```python
from build123d import *

# Parameters (mm, degrees)
PAD_DEPTH       = 20
SKETCH001_R     = 2.6
POCKET_DEPTH    = 25.501
SKETCH002_R     = 5
POCKET001_DEPTH = 21.501
CHAMFER_SIZE    = 4
CHAMFER001_SIZE = 1.5


with BuildPart() as part:
    # Sketch → Pad (new body)
    with BuildSketch(Plane.XY):
        with BuildLine():
            ThreePointArc((-7.433034, 13), (7.5, 14), (-7.433034, 15))
            Line((-7.433034, 15), (-25.5, 15))
            Line((-25.5, 15), (-25.5, 19))
            Line((-25.5, 19), (-10.356158, 19))
            ThreePointArc((8.305538, 21.954121), (-1.798046, 25.358566), (-10.356158, 19))
            Line((25.5, 4), (8.305538, 21.954121))
            Line((25.5, 0), (25.5, 4))
            Line((-25.5, 0), (25.5, 0))
            Line((-25.5, 13), (-25.5, 0))
            Line((-7.433034, 13), (-25.5, 13))
        make_face()
    extrude(amount=PAD_DEPTH)

    # Sketch001 → Pocket (cut, through all)
    with BuildSketch(Plane.XZ):
        with Locations((-16.5, 10)):
            Circle(SKETCH001_R)
        with Locations((16.5, 10)):
            Circle(SKETCH001_R)
    extrude(amount=-POCKET_DEPTH, mode=Mode.SUBTRACT)

    # Sketch002 (on DatumPlane) → Pocket001 (cut, through all)
    with BuildSketch(Plane.XZ.offset(-4)):
        with Locations((16.5, 10)):
            Circle(SKETCH002_R)
    extrude(amount=-POCKET001_DEPTH, mode=Mode.SUBTRACT)

    # Chamfer
    chamfer_edges = [part.edges().sort_by_distance(p)[0] for p in [
        (-25.5, 17, 20),
        (-25.5, 6.5, 20),
        (-25.5, 17, 0),
        (-25.5, 6.5, 0),
        (25.5, 2, 20),
        (25.5, 2, 0),
    ]]
    chamfer(chamfer_edges, length=CHAMFER_SIZE)

    # Chamfer001
    chamfer001_edges = [part.edges().sort_by_distance(p)[0] for p in [
        (7.5, 14, 20),
        (7.5, 14, 0),
        (-1.798046, 25.358566, 20),
        (-15.928079, 19, 20),
        (-23.5, 19, 18),
        (-25.5, 19, 10),
        (-23.5, 19, 2),
        (-15.928079, 19, 0),
        (-1.798046, 25.358566, 0),
        (14.902769, 15.065421, 20),
        (14.902769, 15.065421, 0),
    ]]
    chamfer(chamfer001_edges, length=CHAMFER001_SIZE)


solid = part.part
```
CAD build for the part. Positions are in the model's coordinates, mm. A direction names the side the tool comes from. Coordinates: 2 decimals unless noted, no trailing zeros. Write each loop counter-clockwise with the first axis right and the second up, starting at its lowest first coordinate (ties: lowest second). Pieces come first, ordered by that corner, then holes. Notation, with made-up numbers: (35.25, 61.25) -> (74.25, 61.25) arc R33 cw to (74.25, 94.25) -> close; hole circle Ø3 at (76.25, -37.75). An arc over 180 degrees is marked (long way). Use CSV: the item, a comma, the result in double quotes. Start each with the question number.
Item 1: Band-saw the part on C-C, the plane z = 10. Write the cut outline in (x, y), plus the area to 3 significant figures.
Item 2: Two-plate mould, pull along Y, no slides. Class faces 4 (the flat face through (0, 0, 10)), 5 (the flat face through (-14, 15, 8)), 6 (the conical face through (-1.927, 24.078, 0.26)), 7 (the conical face through (8, 14, 19)): +Y half, -Y half, draft (parallel to the pull), parting line (faces both ways), or undercut.
Item 3: Tool access for faces 1 (the flat face through (-15.5, 18.3, 0.8)), 2 (the cylindrical face through (11.505, 9.665, 10.22)), 3 (the flat face through (-15.5, 18.3, 19.2)): list every direction of +Z, -Z, +X, -X, +Y, -Y with a clear straight run to the whole face (end or side of a thin tool).
Item 4: Band-saw the part on A-A, the plane x = 0. Write the cut outline in (y, z), plus the area to 3 significant figures.
Item 5: Band-saw the part on B-B, the plane y = 2.5. Write the cut outline in (x, z), plus the area to 3 significant figures.
Item 6: Band-saw the part on D-D, the plane x = -16.5. Write the cut outline in (y, z), plus the area to 3 significant figures.
Item 7: Drop flat-ended pins along their axis: P1, Ø1, axis at y = 12.5, z = 7, coming from the +X side; P2, Ø7, axis at x = -14, z = 6.5, coming from the +Y side; P3, Ø8, axis at y = 12.5, z = 12, coming from the +X side. Give the stop position or say it passes through.
Item 8: Wall check: probe 1 along X at (y, z) = (8.25, 6.25); probe 2 along Z at (x, y) = (16.5, 1.65); probe 3 along X at (y, z) = (10.5, 8). Give the ranges that are in metal, low to high.
Response values:
1,outline,"(-25.5, 0) -> (-19.1, 0) -> (-19.1, 13) -> (-25.5, 13) -> close; (-25.5, 15) -> (-19.1, 15) -> (-19.1, 19) -> (-24, 19) -> (-25.5, 17.5) -> close; (-13.9, 0) -> (13.9, 0) -> (13.9, 4) -> (11.5, 4) -> (11.5, 18.62) -> (8.31, 21.95) arc R11.5 ccw to (-10.36, 19) -> (-13.9, 19) -> (-13.9, 15) -> (-7.43, 15) arc R7.5 cw (long way) to (-7.43, 13) -> (-13.9, 13) -> close; (19.1, 0) -> (25.5, 0) -> (25.5, 4) -> (21.5, 8.18) -> (21.5, 4) -> (19.1, 4) -> close"
1,area,"541 mm2"
2,face 4,"-Y half"
2,face 5,"undercut"
2,face 6,"+Y half"
2,face 7,"undercut"
3,face 1,"-Z, -X, +Y"
3,face 2,"+Y"
3,face 3,"+Z, -X, +Y"
4,outline,"(0, 0) -> (5, 0) -> (6.5, 1.5) -> (6.5, 18.5) -> (5, 20) -> (0, 20) -> close; (21.5, 1.5) -> (23, 0) -> (24, 0) -> (25.5, 1.5) -> (25.5, 18.5) -> (24, 20) -> (23, 20) -> (21.5, 18.5) -> close"
4,area,"203 mm2"
5,outline,"(-25.5, 4) -> (-21.5, 0) -> (21.5, 0) -> (25.5, 4) -> (25.5, 16) -> (21.5, 20) -> (-21.5, 20) -> (-25.5, 16) -> close; hole circle Ø5.2 at (-16.5, 10); hole circle Ø5.2 at (16.5, 10)"
5,area,"946 mm2"
6,outline,"(0, 0) -> (13, 0) -> (13, 7.4) -> (0, 7.4) -> close; (0, 12.6) -> (13, 12.6) -> (13, 20) -> (0, 20) -> close; (15, 0) -> (17.5, 0) -> (19, 1.5) -> (19, 7.4) -> (15, 7.4) -> close; (15, 12.6) -> (19, 12.6) -> (19, 18.5) -> (17.5, 20) -> (15, 20) -> close"
6,area,"249 mm2"
7,P1,"stops at x = 12.93"
7,P2,"stops at y = 19"
7,P3,"stops at x = 21.19"
8,probe 1,"x = -25.5 to -4.82, 4.82 to 13.19, 19.81 to 21.43"
8,probe 2,"z = 0 to 7.4, 12.6 to 20"
8,probe 3,"x = -25.5 to -18.16, -14.84 to -6.63, 6.63 to 11.92"
